Read the model definition and answer for the solid it produces. Units are mm, in the model's axes. A direction names the side the tool comes from. Coordinates: 2 decimals unless noted, no trailing zeros. Loops run counter-clockwise (first coordinate to the right, second up) from the corner with the lowest first, then second, coordinate; pieces in that order, holes last. Notation, with made-up numbers: (83, -23) -> (99, -23) arc R14 cw to (99, -1) -> close; hole circle Ø11 at (57.5, 5.5). An arc over 180 degrees is marked (long way). Answer as a JSON object with one key per item and string values. Group by question number.
1) Which of the six approach directions +Z, -Z, +X, -X, +Y, -Y give full straight-line access (tool end or side, diameter ignored) to faces 1 (the face through (-0.691, -3.112, 0.188)), 2 (the face through (-0.99, 1.74, 2.01))?
2) Section B-B, the plane z = -4 is taken. Give the vertices of the cut face in (x, y), plus the area to 3 significant figures.
3) Consider probe 1 along Z at (x, y) = (-0.75, 0.5); probe 2 along Y at (x, z) = (-2.25, -5); probe 3 along Z at (x, y) = (2, 4.25). Determine where each line is inside the solid, lowest interval first. Write a range as [from, to].
4) Determine the mould class of faces 3 (the face through (2.86, -0.9, -6.26)), 4 (the face through (3, 0, 3)), 5 (the face through (2, 0, 2)) for opening direction Y: released by +Y, released by -Y, zero draft, split by the parting line, or undercut.
5) Flat-ended cylindrical pins translate along their axes: P1, Ø0.6, axis at y = 0, z = 2.5, coming from the +X side; P2, Ø1.6, axis at y = 0, z = 2, coming from the -X side; P3, Ø1, axis at y = 1, z = -3.5, coming from the -X side. Find the tip coordinate at first contact, or state that the pin passes through.
from build123d import *

# Parameters (mm, degrees)
SKETCH1_R           = 6
BOSS_EXTRUDE1_DEPTH = 3
SKETCH2_R           = 3
BOSS_EXTRUDE2_DEPTH = 13
CHAMFER1_SIZE       = 0.3
CUT_EXTRUDE1_DEPTH  = 2
CHAMFER2_SIZE       = 3


with BuildPart() as part:
    # Sketch1 → Boss-Extrude1 (new body)
    with BuildSketch(Plane.XY):
        Circle(SKETCH1_R)
    extrude(amount=BOSS_EXTRUDE1_DEPTH)

    # Sketch2 → Boss-Extrude2 (add)
    with BuildSketch(Plane(origin=(0, 0, 0), x_dir=(-1, 0, 0), z_dir=(0, 0, -1))):
        with Locations(Location((0, 0, 0), (0, 0, 180))):
            Circle(SKETCH2_R)
    extrude(amount=BOSS_EXTRUDE2_DEPTH)

    # Chamfer1
    chamfer1_edges = [part.edges().sort_by_distance(p)[0] for p in [
        (-3, 0, -13),
    ]]
    chamfer(chamfer1_edges, length=CHAMFER1_SIZE)

    # Sketch3 → Cut-Extrude1 (cut)
    with BuildSketch(Plane.XY.offset(3)):
        Polygon((0, 2.309401077), (-2, 1.154700538), (-2, -1.154700538), (0, -2.309401077), (2, -1.154700538), (2, 1.154700538), align=None)
    extrude(amount=-CUT_EXTRUDE1_DEPTH, mode=Mode.SUBTRACT)

    # Chamfer2
    chamfer2_edges = [part.edges().sort_by_distance(p)[0] for p in [
        (-6, 0, 0),
    ]]
    chamfer(chamfer2_edges, length=CHAMFER2_SIZE - 0.0001)  # a hair under: the kernel refuses the full size


solid = part.part
Determined:
{
 "1": {"face 1": "-Z", "face 2": "+Z"},
 "2": {"outline": "circle Ø6 at (0, 0)", "area": "28.3 mm²"},
 "3": {"probe 1": "[-13, 1]", "probe 2": "[-1.98, 1.98]", "probe 3": "[1.7, 3]"},
 "4": {"face 3": "split by the parting line", "face 4": "zero draft", "face 5": "undercut"},
 "5": {"P1": "x = 5.8", "P2": "x = -5.8", "P3": "x = -2.96"}
}
